The listing builds one solid part. Answer for the finished solid, in the listing's coordinates (mm). Round coordinates to 2 decimals unless told otherwise and drop trailing zeros. Loops run counter-clockwise (first coordinate to the right, second up) from the corner with the lowest first, then second, coordinate; pieces in that order, holes last. Notation, with made-up numbers: (47, -10.5) -> (63, -10.5) arc R21 ccw to (63, 15.5) -> close; hole circle Ø5 at (-33.5, -25.75). An arc over 180 degrees is marked (long way). Use a Markdown table: item, result. Add a question column.
Q1. Consider line 1 (Y direction, x = -42, z = 4.6); line 2 (Y direction, x = -34.5, z = 4.4); line 3 (X direction, y = 58, z = 1.6). Determine where each line is inside the solid, lowest interval first.
Q2. Section B-B on y = 12.5 is taken. Give the vertices of the cut face in (x, z).
Q3. Section A-A on y = 103 is taken. Give the vertices of the cut face in (x, z), then the cut area to 3 significant figures.
Q4. Section D-D on z = 3.35 is taken. Give the number of separate pieces and of enclosed holes in the cut face, then the cut area to 3 significant figures.
Q5. Section C-C on x = -27 is taken. Give the vertices of the cut face in (y, z).
Q6. Given pin 1 Ø2 at (x, z) = (-47, 3.5) entering from +Y, flat-ended and moving along its own axis, determine where the tip first touches the part or whether it passes through.
from build123d import *

# Parameters (mm, degrees)
SKETCH1_R           = 1.65
SKETCH1_W           = 30
SKETCH1_H           = 5
BOSS_EXTRUDE1_DEPTH = 5
CUT_EXTRUDE1_DEPTH  = 6
FILLET1_R           = 10


with BuildPart() as part:
    # Sketch1 → Boss-Extrude1 (new body)
    with BuildSketch(Plane.XY):
        Polygon((-52.5, 172), (-22.5, 172), (-22.5, 180), (-7.5, 180), (-7.5, 172), (-2.5, 172), (-2.5, 0), (-72.5, 0), (-72.5, 172), (-67.5, 172), (-67.5, 180), (-52.5, 180), align=None)
        with Locations((-62.5, 12.5)):
            Circle(SKETCH1_R, mode=Mode.SUBTRACT)
        with Locations((-12.5, 12.5)):
            Circle(SKETCH1_R, mode=Mode.SUBTRACT)
        with Locations((-37.5, 12.5)):
            Rectangle(SKETCH1_W, SKETCH1_H, mode=Mode.SUBTRACT)
        with BuildLine():
            Line((-32.5, 147), (-42.5, 147))
            ThreePointArc((-42.5, 147), (-49.571067812, 144.071067812), (-52.5, 137))
            Line((-52.5, 137), (-52.5, 57))
            ThreePointArc((-52.5, 57), (-49.571067812, 49.928932188), (-42.5, 47))
            Line((-42.5, 47), (-32.5, 47))
            ThreePointArc((-32.5, 47), (-25.428932188, 49.928932188), (-22.5, 57))
            Line((-22.5, 57), (-22.5, 137))
            ThreePointArc((-22.5, 137), (-25.428932188, 144.071067812), (-32.5, 147))
        make_face(mode=Mode.SUBTRACT)
    extrude(amount=BOSS_EXTRUDE1_DEPTH)

    # Sketch2 → Cut-Extrude1 (cut, through all)
    with BuildSketch(Plane.XY.offset(5)):
        Polygon((-35.85, 172), (-35.85, 168), (-34, 168), (-34, 165.8), (-35.85, 165.8), (-35.85, 163.8), (-39.15, 163.8), (-39.15, 165.8), (-41, 165.8), (-41, 168), (-39.15, 168), (-39.15, 172), align=None)
    extrude(amount=-CUT_EXTRUDE1_DEPTH, mode=Mode.SUBTRACT)

    # Fillet1
    fillet1_edges = [part.edges().sort_by_distance(p)[0] for p in [
        (-2.5, 0, 2.5),
        (-72.5, 0, 2.5),
    ]]
    fillet(fillet1_edges, radius=FILLET1_R)


solid = part.part
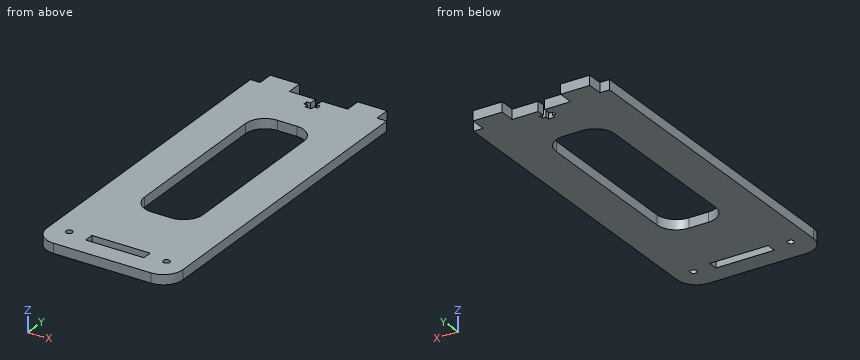
Checked values:
| question | item | result |
|---|---|---|
| 1 | line 1 | y = 0 to 10, 15 to 47, 147 to 172 |
| 1 | line 2 | y = 0 to 10, 15 to 47, 147 to 165.8, 168 to 172 |
| 1 | line 3 | x = -72.5 to -52.5, -22.5 to -2.5 |
| 2 | outline | (-72.5, 0) -> (-64.15, 0) -> (-64.15, 5) -> (-72.5, 5) -> close; (-60.85, 0) -> (-52.5, 0) -> (-52.5, 5) -> (-60.85, 5) -> close; (-22.5, 0) -> (-14.15, 0) -> (-14.15, 5) -> (-22.5, 5) -> close; (-10.85, 0) -> (-2.5, 0) -> (-2.5, 5) -> (-10.85, 5) -> close |
| 3 | outline | (-72.5, 0) -> (-52.5, 0) -> (-52.5, 5) -> (-72.5, 5) -> close; (-22.5, 0) -> (-2.5, 0) -> (-2.5, 5) -> (-22.5, 5) -> close |
| 3 | area | 200 mm2 |
| 4 | separate pieces | 1 |
| 4 | enclosed holes | 4 |
| 4 | area | 9,120 mm2 |
| 5 | outline | (0, 0) -> (10, 0) -> (10, 5) -> (0, 5) -> close; (15, 0) -> (48.65, 0) -> (48.65, 5) -> (15, 5) -> close; (145.35, 0) -> (172, 0) -> (172, 5) -> (145.35, 5) -> close |
| 6 | pin 1 | stops at y = 172 |
